from build123d import *

# Parameters (mm, degrees)
F0_R          = 12.5
F0_R_2        = 5.5
F0_R_3        = 16.5
F1_DEPTH      = 1.6
F0_R_4        = 4.25
F2_DEPTH      = 19
F2_DEPTH_BACK = 1.6
F3_R          = 4
F4_DEPTH      = 18
F5_R          = 4.25
F6_DEPTH      = 18


with BuildPart() as f1:
    # F0 (on Right) → F1 (new body)
    with BuildSketch(Plane.YZ):
        with BuildLine():
            Line((-402, 0), (0, 0))
            Line((0, 0), (0, 51))
            ThreePointArc((0, 51), (-0.2928932188, 51.7071067812), (-1, 52))
            Line((-1, 52), (-206, 52))
            Line((-206, 52), (-401.2095290887, 10.1693866238))
            ThreePointArc((-401.2095290887, 10.1693866238), (-401.777666088, 9.8202617548), (-402, 9.1915842098))
            Line((-402, 9.1915842098), (-402, 0))
        make_face()
        with Locations((-231.9873586528, 25)):
            Circle(F0_R, mode=Mode.SUBTRACT)
        with Locations((-192.5874, 18)):
            Circle(F0_R_2, mode=Mode.SUBTRACT)
        with Locations((-143, 26.5)):
            Circle(F0_R_3, mode=Mode.SUBTRACT)
        with Locations((-45, 26.5)):
            Circle(F0_R_3, mode=Mode.SUBTRACT)
        with Locations((-91, 42.5)):
            Circle(F0_R_2, mode=Mode.SUBTRACT)
    extrude(amount=F1_DEPTH)

    # F0 (on Right) → F2 (join, two sides)
    with BuildSketch(Plane.YZ) as f2_sk:
        with Locations((-91, 42.5)):
            Circle(F0_R_2)
        with Locations((-91, 42.5)):
            Circle(F0_R_4, mode=Mode.SUBTRACT)
        with Locations((-192.5874, 18)):
            Circle(F0_R_2)
        with Locations((-192.5874, 18)):
            Circle(F0_R_4, mode=Mode.SUBTRACT)
        with Locations((-91, 42.5)):
            Circle(F0_R_4)
        with Locations((-192.5874, 18)):
            Circle(F0_R_4)
    extrude(amount=-F2_DEPTH)
    extrude(f2_sk.sketch, amount=F2_DEPTH_BACK)

    # F3 (on face) → F4 (cut)
    with BuildSketch(Plane(origin=(-19, 0, 0), x_dir=(0, -1, 0), z_dir=(-1, 0, 0))):
        with Locations((91, 42.5)):
            Circle(F3_R)
    extrude(amount=-F4_DEPTH, mode=Mode.SUBTRACT)

    # F5 (on face) → F6 (cut)
    with BuildSketch(Plane(origin=(-19, 0, 0), x_dir=(0, -1, 0), z_dir=(-1, 0, 0))):
        with Locations((192.5874, 18)):
            Circle(F5_R)
    extrude(amount=-F6_DEPTH, mode=Mode.SUBTRACT)


solid = f1.part
Geometry: final body of the model. Coordinates: model frame, mm. A direction names the side the tool comes from. Round coordinates to 2 decimals unless told otherwise and drop trailing zeros. Loops run counter-clockwise (first coordinate to the right, second up) from the corner with the lowest first, then second, coordinate; pieces in that order, holes last.
Q1. Material intervals for L1, parallel to X at y = -152, z = 4; L2, parallel to Z at x = -4.5, y = -196; L3, parallel to Y at x = -3.5, z = 16.5, sorted ascending.
Q2. Section B-B on z = 32. Return loops of the section in (x, y).
Q3. Access query for faces 1 (the cylindrical face through (0.789, -159.484, 27.225)), 2 (the cylindrical face through (-9.367, -96.495, 42.742)). Directions: +Z, -Z, +X, -X, +Y, -Y. A direction counts if a zero-diameter tool reaches every point of the face in a straight line with its end or side. Return the directions, or none.
Q4. Section D-D on z = 4.5. Return loops of the section in (x, y).
Q5. Section C-C on y = -91. Return loops of the section in (x, z).
Q6. Section A-A on x = -12.5. Return loops of the section in (y, z), plus the area to 3 significant figures.
Q7. Pull-direction query (Y, two-part tool) for faces 3 (the flat face through (-19, -190, 14)), 4 (the flat face through (-1, -193, 18)), 5 (the flat face through (0.789, -302.238, 31.378)); classes: released by +Y, released by -Y, zero draft, split by the parting line, or undercut.
Q8. Pin query (flat end, axial travel): P1, Ø4, axis at y = -193.5, z = 18, coming from the -X side; P2, Ø10, axis at x = -3, y = -360.5, coming from the +Z side; P3, Ø1, axis at x = -2, z = 41, coming from the +Y side; P4, Ø8, axis at x = -1.5, z = 20, coming from the +Y side. Return the tip coordinate at first contact, or that it passes through.
Evaluation:
1. L1: x = 0 to 1.6
1. L2: z = 13.69 to 15.47, 20.53 to 22.31
1. L3: y = -197.88 to -196.56, -188.61 to -187.3
2. outline: (0, -299.33) - (1.6, -299.33) - (1.6, -242.34) - (0, -242.34) - close; (0, -221.63) - (1.6, -221.63) - (1.6, -158.56) - (0, -158.56) - close; (0, -127.44) - (1.6, -127.44) - (1.6, -60.56) - (0, -60.56) - close; (0, -29.44) - (1.6, -29.44) - (1.6, 0) - (0, 0) - close
3. face 1: +X, -X
3. face 2: -X
4. outline: (0, -402) - (1.6, -402) - (1.6, 0) - (0, 0) - close
5. outline: (-19, 37) - (0, 37) - (0, 0) - (1.6, 0) - (1.6, 52) - (0, 52) - (0, 48) - (-19, 48) - (-19, 46.5) - (-1, 46.5) - (-1, 38.5) - (-19, 38.5) - close
6. outline: circle Ø11 at (-192.59, 18); circle Ø11 at (-91, 42.5); hole circle Ø8.5 at (-192.59, 18); hole circle Ø8 at (-91, 42.5)
6. area: 83.1 mm2
7. face 3: zero draft
7. face 4: undercut
7. face 5: released by -Y
8. P1: stops at x = -1
8. P2: stops at z = 19.75
8. P3: stops at y = -85.59
8. P4: stops at y = 0
